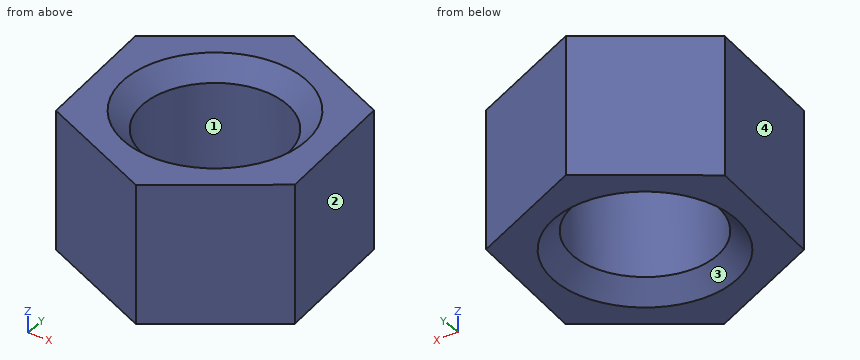
```python
from build123d import *

# Parameters (mm, degrees)
BOSS_EXTRUDE1_DEPTH = 15
SKETCH2_R           = 7.75
CUT_EXTRUDE1_DEPTH  = 25.526787522
CHAMFER1_SIZE       = 2


with BuildPart() as part:
    # Sketch1 → Boss-Extrude1 (new body)
    with BuildSketch(Plane.XY):
        Polygon((13.017705446, -6.234795766), (11.908344244, 8.156265732), (-1.109361202, 14.391061499), (-13.017705446, 6.234795766), (-11.908344244, -8.156265732), (1.109361202, -14.391061499), align=None)
    extrude(amount=BOSS_EXTRUDE1_DEPTH)

    # Sketch2 → Cut-Extrude1 (cut, through all)
    with BuildSketch(Plane(origin=(0, 0, 0), x_dir=(-1, 0, 0), z_dir=(0, 0, -1))):
        Circle(SKETCH2_R)
    extrude(amount=-CUT_EXTRUDE1_DEPTH, mode=Mode.SUBTRACT)

    # Chamfer1
    chamfer1_edges = [part.edges().sort_by_distance(p)[0] for p in [
        (7.75, 0, 15),
        (7.75, 0, 0),
    ]]
    chamfer(chamfer1_edges, length=CHAMFER1_SIZE)


solid = part.part
```
Check sheet for the modelled part. Datum: model origin and axes. Units: mm. Face numbers are marked on the shaded views. Round coordinates to 2 decimals unless told otherwise and drop trailing zeros. Loops run counter-clockwise (first coordinate to the right, second up) from the corner with the lowest first, then second, coordinate; pieces in that order, holes last. Notation, with made-up numbers: (40.5, 0) - (99.5, 0) arc R20 cw to (99.5, 21) - close; hole circle Ø11 at (-4.75, 83.25). An arc over 180 degrees is marked (long way). Write item = value, one per line. Start each with the question number.
Q1. Section check A-A (z = 8.5). Record the boundary of the cut face in (x, y), plus the area to 3 significant figures.
Q2. Section check B-B (x = 0). Record the boundary of the cut face in (y, z), plus the area to 3 significant figures.
Q3. Section check D-D (z = 13.75). Record the boundary of the cut face in (x, y), plus the area to 3 significant figures.
Q4. Release check for a two-part mould opening along X. For the marked faces 1, 2, 3 and 4 record: pulls with the +X half, pulls with the -X half, needs draft (parallel to the pull), parting line crosses it, or undercut.
Q5. Depth check by flat-ended pin: P1, Ø4, axis at x = 2.5, y = 7, coming from the +Z side; P2, Ø8, axis at x = -6, z = 12, coming from the +Y side; P3, Ø3, axis at y = -2, z = 2.5, coming from the -X side. Enter the tip coordinate at first touch or a pass-through.
Q6. Section check C-C (y = 0). Record the boundary of the cut face in (x, z), plus the area to 3 significant figures.
Q7. Thickness scan on L1, parallel to Y at x = 1, z = 5.5; L2, parallel to Y at x = -6, z = 12; L3, parallel to X at y = -7, z = 1.75. Record the ranges inside material, lowest first.
Derived:
q1.outline = (-13.02, 6.23) - (-11.91, -8.16) - (1.11, -14.39) - (13.02, -6.23) - (11.91, 8.16) - (-1.11, 14.39) - close; hole circle Ø15.5 at (0, 0)
q1.area = 353 mm^2
q2.outline = (-13.86, 0) - (-9.75, 0) - (-7.75, 2) - (-7.75, 13) - (-9.75, 15) - (-13.86, 15) - close; (7.75, 2) - (9.75, 0) - (13.86, 0) - (13.86, 15) - (9.75, 15) - (7.75, 13) - close
q2.area = 175 mm^2
q3.outline = (-13.02, 6.23) - (-11.91, -8.16) - (1.11, -14.39) - (13.02, -6.23) - (11.91, 8.16) - (-1.11, 14.39) - close; hole circle Ø17 at (0, 0)
q3.area = 314 mm^2
q4.face_1 = undercut
q4.face_2 = pulls with the +X half
q4.face_3 = undercut
q4.face_4 = pulls with the -X half
q5.P1 = 14.68
q5.P2 = 13.78
q5.P3 = -12.5
q6.outline = (-12.54, 0) - (-9.75, 0) - (-7.75, 2) - (-7.75, 13) - (-9.75, 15) - (-12.54, 15) - close; (7.75, 2) - (9.75, 0) - (12.54, 0) - (12.54, 15) - (9.75, 15) - (7.75, 13) - close
q6.area = 136 mm^2
q7.L1 = -14.34 to -7.69, 7.69 to 13.38
q7.L2 = -10.99 to -4.91, 4.91 to 11.04
q7.L3 = -12 to -3.87, 3.87 to 11.9
